```python
from build123d import *

# Parameters (mm, degrees)
SKETCH_1_W          = 100
SKETCH_1_H          = 40
EXTRUDE_1_DEPTH     = 10
EXTRUDE_2_DEPTH     = 10
SKETCH_4_R          = 12.5
CUT_EXTRUDE_1_DEPTH = 5
SKETCH_5_R          = 6
CUT_EXTRUDE_2_DEPTH = 5
SKETCH_6_W          = 30
SKETCH_6_H          = 5
CUT_EXTRUDE_3_DEPTH = 85.409715081
FILLET_1_R          = 8
FILLET_2_R          = 3
SKETCH_7_R          = 4
CUT_EXTRUDE_5_DEPTH = 71.178344238


with BuildPart() as part:
    # Эскиз1 → Бобышка-Вытянуть1 (new body)
    with BuildSketch(Plane.XY):
        Rectangle(SKETCH_1_W, SKETCH_1_H)
    extrude(amount=EXTRUDE_1_DEPTH)

    # Эскиз2 → Бобышка-Вытянуть2 (add)
    with BuildSketch(Plane.XZ.offset(20)):
        with BuildLine():
            Line((-20, 0), (-20, 35))
            ThreePointArc((-20, 35), (0, 55), (20, 35))
            Line((20, 35), (20, 0))
            Line((20, 0), (-20, 0))
        make_face()
    extrude(amount=-EXTRUDE_2_DEPTH)

    # Эскиз4 → Вырез-Вытянуть1 (cut)
    with BuildSketch(Plane.XZ.offset(20)):
        with Locations((0, 35)):
            Circle(SKETCH_4_R)
    extrude(amount=-CUT_EXTRUDE_1_DEPTH, mode=Mode.SUBTRACT)

    # Эскиз5 → Вырез-Вытянуть2 (cut)
    with BuildSketch(Plane.XZ.offset(15)):
        with Locations((0, 35)):
            Circle(SKETCH_5_R)
    extrude(amount=-CUT_EXTRUDE_2_DEPTH, mode=Mode.SUBTRACT)

    # Эскиз6 → Вырез-Вытянуть3 (cut, through all)
    with BuildSketch(Plane.XZ.offset(20)):
        with Locations((0, 2.5)):
            Rectangle(SKETCH_6_W, SKETCH_6_H)
    extrude(amount=-CUT_EXTRUDE_3_DEPTH, mode=Mode.SUBTRACT)

    # Скругление1
    # the kernel refuses this fillet: 8 mm, written as the material it adds along each edge
    with BuildSketch(Plane(origin=(-15, -20, 5), x_dir=(1, 0, 0), z_dir=(0, 1, 0))) as fillet_1_piece_1:
        with BuildLine():
            CenterArc((7.416198487, 8), FILLET_1_R, 202.024312837, 67.975687163)
            Line((0, 5), (0, 0))
            Line((0, 0), (7.416198487, 0))
        make_face()
    extrude(amount=40)
    with BuildSketch(Plane(origin=(15, -20, 5), x_dir=(0, 0, -1), z_dir=(0, 1, 0))) as fillet_1_piece_2:
        with BuildLine():
            CenterArc((8, 7.416198487), FILLET_1_R, 180, 67.975687163)
            Line((0, 7.416198487), (0, 0))
            Line((0, 0), (5, 0))
        make_face()
    extrude(amount=40)
    # the kernel refuses this fillet: 8 mm, written as the material it takes off along each edge
    with BuildSketch(Plane(origin=(50, -20, -20), x_dir=(-1, 0, 0), z_dir=(0, 0, 1)), Plane(origin=(50, 20, -20), x_dir=(0, -1, 0), z_dir=(0, 0, 1))) as fillet_1_2_piece_1:
        with BuildLine():
            CenterArc((FILLET_1_R, -FILLET_1_R), FILLET_1_R, 90, 90)
            Line((0, -FILLET_1_R), (0, 0))
            Line((0, 0), (FILLET_1_R, 0))
        make_face()
    extrude(amount=50, mode=Mode.SUBTRACT)
    with BuildSketch(Plane(origin=(-50, -20, -20), x_dir=(1, 0, 0), z_dir=(0, 0, 1)), Plane(origin=(-50, 20, -20), x_dir=(0, -1, 0), z_dir=(0, 0, 1))) as fillet_1_2_piece_2:
        with BuildLine():
            CenterArc((FILLET_1_R, FILLET_1_R), FILLET_1_R, 180, 90)
            Line((0, FILLET_1_R), (0, 0))
            Line((0, 0), (FILLET_1_R, 0))
        make_face()
    extrude(amount=50, mode=Mode.SUBTRACT)

    # Скругление2
    fillet_2_edges = [part.edges().sort_by_distance(p)[0] for p in [
        (31, -20, 10),
        (-20, -15, 10),
        (-20, -20, 22.5),
        (0, -20, 55),
        (20, -15, 10),
        (0, -10, 10),
        (20, -20, 22.5),
        (50, 0, 10),
        (-31, -20, 10),
        (0, 20, 10),
        (-50, 0, 10),
        (47.656854249, 17.656854249, 10),
        (-47.656854249, 17.656854249, 10),
        (-47.656854249, -17.656854249, 10),
        (47.656854249, -17.656854249, 10),
    ]]
    fillet(fillet_2_edges, radius=FILLET_2_R)

    # Эскиз7 → Вырез-Вытянуть5 (cut, through all)
    with BuildSketch(Plane.XY.offset(10)):
        with Locations((-42, 12)):
            Circle(SKETCH_7_R)
        with Locations(Location((42, 12, 0), (0, 0, 180))):
            Circle(SKETCH_7_R)
    extrude(amount=-CUT_EXTRUDE_5_DEPTH, mode=Mode.SUBTRACT)


solid = part.part
```
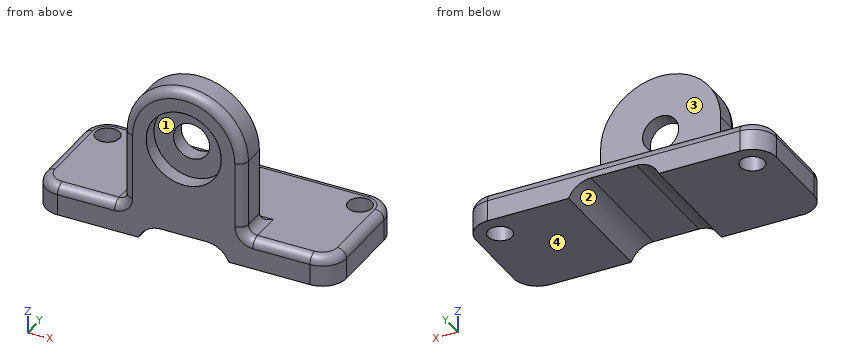
Read the model definition and answer for the solid it produces. Units are mm, in the model's axes. Face numbers are marked on the shaded views. A direction names the side the tool comes from. Coordinates: 2 decimals unless noted, no trailing zeros. Write each loop counter-clockwise with the first axis right and the second up, starting at its lowest first coordinate (ties: lowest second). Pieces come first, ordered by that corner, then holes. Notation, with made-up numbers: (-31.5, 58.5) -> (13.5, 58.5) arc R29 cw to (13.5, 90.5) -> close; hole circle Ø6 at (4.5, -17.75). An arc over 180 degrees is marked (long way). Write item = value, one per line.
(1) Section D-D on x = 39 is taken. Write down the section's boundary in (y, z).
From the geometry:
outline = (-20, 0) -> (9.35, 0) -> (9.35, 10) -> (-17, 10) arc R3 ccw to (-20, 7) -> close; (14.65, 0) -> (20, 0) -> (20, 7) arc R3 ccw to (17, 10) -> (14.65, 10) -> close
(2) Given pin 1 Ø12 at (x, y) = (-30, 4) entering from +Z; pin 2 Ø10 at (x, y) = (-11, -6.5) entering from +Z; pin 3 Ø5 at (x, y) = (42, 12) entering from -Z; pin 4 Ø10 at (x, y) = (20, -8) entering from +Z, each flat-ended and moving along its own axis, determine where each tip first touches the part or whether it passes through.
From the geometry:
pin_1 = 10
pin_2 = 53.57
pin_3 = through
pin_4 = 47.74
(3) Section C-C on y = -3 is taken. Write down the section's boundary in (x, z), plus the area to 3 significant figures.
From the geometry:
outline = (-50, 0) -> (-15, 0) arc R8 cw to (-7.58, 5) -> (7.58, 5) arc R8 cw to (15, 0) -> (50, 0) -> (50, 7) arc R3 ccw to (47, 10) -> (-47, 10) arc R3 ccw to (-50, 7) -> close
area = 867 mm2
(4) Section B-B on z = 33 is taken. Write down the section's boundary in (x, y), plus the area to 3 significant figures.
From the geometry:
outline = (-20, -17) arc R3 ccw to (-17, -20) -> (-12.34, -20) -> (-12.34, -15) -> (-5.66, -15) -> (-5.66, -10) -> (-20, -10) -> close; (5.66, -15) -> (12.34, -15) -> (12.34, -20) -> (17, -20) arc R3 ccw to (20, -17) -> (20, -10) -> (5.66, -10) -> close
area = 216 mm2
(5) Which of the six approach directions +Z, -Z, +X, -X, +Y, -Y give full straight-line access (tool end or side, diameter ignored) to the marked faces 1, 2, 3 and 4?
From the geometry:
face_1 = -Y
face_2 = -Z, +Y, -Y
face_3 = +Z, +X, -X, +Y
face_4 = -Z, +X, -X, +Y, -Y
(6) Section A-A on x = 0 is taken. Write down the section's boundary in (y, z), plus the area to 3 significant figures.
From the geometry:
outline = (-20, 5) -> (20, 5) -> (20, 7) arc R3 ccw to (17, 10) -> (-7, 10) arc R3 cw to (-10, 13) -> (-10, 29) -> (-15, 29) -> (-15, 22.5) -> (-20, 22.5) -> close; (-20, 47.5) -> (-15, 47.5) -> (-15, 41) -> (-10, 41) -> (-10, 55) -> (-17, 55) arc R3 ccw to (-20, 52) -> close
area = 463 mm2
(7) Straight lines are drawn through the part: L1, parallel to Z at x = 0, y = -13; L2, parallel to Y at x = -42, z = 2; L3, parallel to Y at x = 0.5, z = 17.5. For each, find the intervals that lie inside material, in ascending order. Write a range as from..to.
From the geometry:
L1 = 5..29, 41..55
L2 = -20..8, 16..20
L3 = -20..-10
